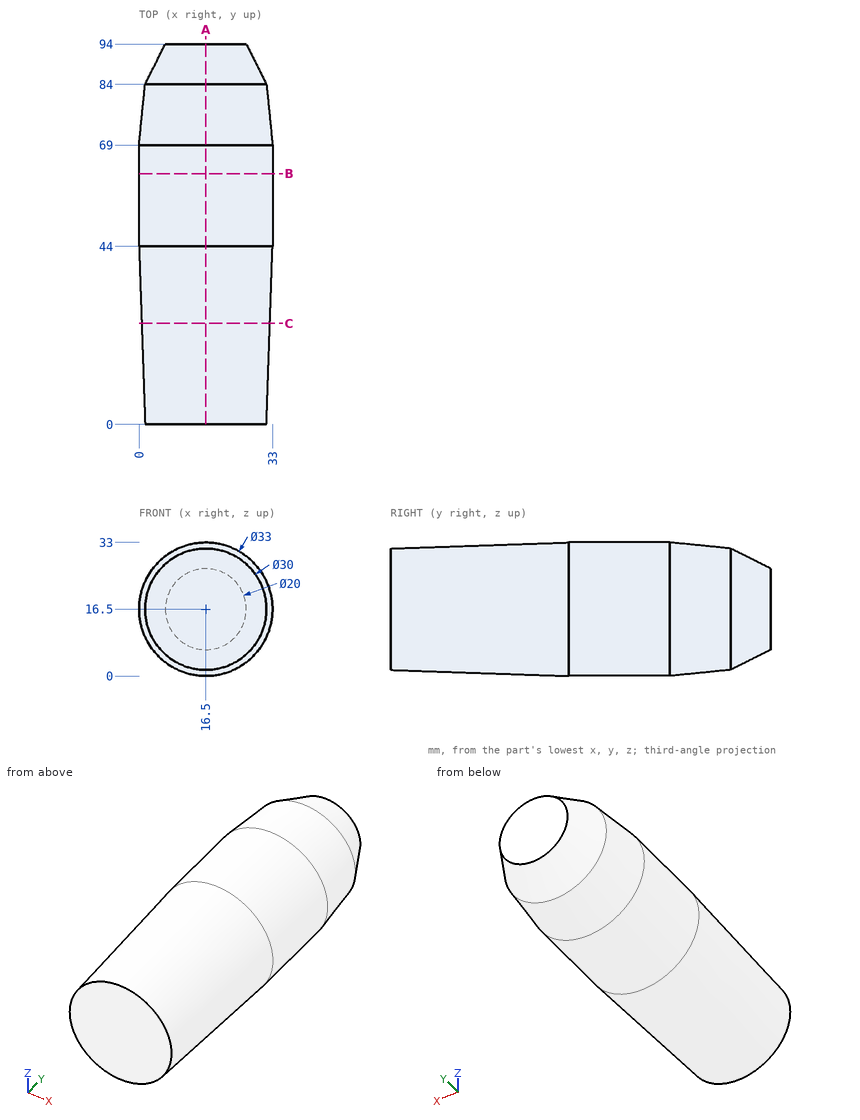
Input: dimensioned drawing with shaded views. Units: mm. Origin: part minimum x, y, z. Round coordinates to 2 decimals unless told otherwise and drop trailing zeros. Order: outer loops, then holes, each group sorted by start corner. A loop starts at its lowest first (then second) coordinate and runs counter-clockwise, first axis right, second up. Notation, with made-up numbers: M -39,30 L 11,30 A22 ccw 11,38 Z; hole C -9.5,86.25 d10. An arc over 180 degrees is marked long. Use one line per item in the form item = value. Start each with the question number.
Q1. Cut plane B-B (y = 62). Return loops of the section in (x, z), and give its area (3 significant figures).
Q2. Pin query (flat end, axial travel): pin 1 Ø3 at (y, z) = (38.5, 13) entering from +X; pin 2 Ø1 at (y, z) = (34.5, 20.5) entering from +X; pin 3 Ø2 at (y, z) = (25, 25.5) entering from +X. Return the tip coordinate at first contact, or that it passes through.
Q3. Cut plane C-C (y = 25). Return loops of the section in (x, z), and give its area (3 significant figures).
Q4. Cut plane A-A (x = 16.5). Return loops of the section in (y, z).
Q5. Material intervals for line 1 (X direction, y = 8, z = 12); line 2 (X direction, y = 58, z = 19.5); line 3 (Z direction, x = 30, y = 82), sorted ascending. Write a range as [from, to].
Geometry results:
q1.outline = C 16.5,16.5 d33
q1.area = 855 mm^2
q2.pin_1 = 32.7
q2.pin_2 = 32.29
q2.pin_3 = 30.19
q3.outline = C 16.5,16.5 d31.7
q3.area = 789 mm^2
q4.outline = M 0,1.5 L 44,0 L 69,0 L 84,1.5 L 94,6.5 L 94,26.5 L 84,31.5 L 69,33 L 44,33 L 0,31.5 Z
q5.line_1 = [1.91, 31.09]
q5.line_2 = [0.28, 32.72]
q5.line_3 = [9.52, 23.48]
